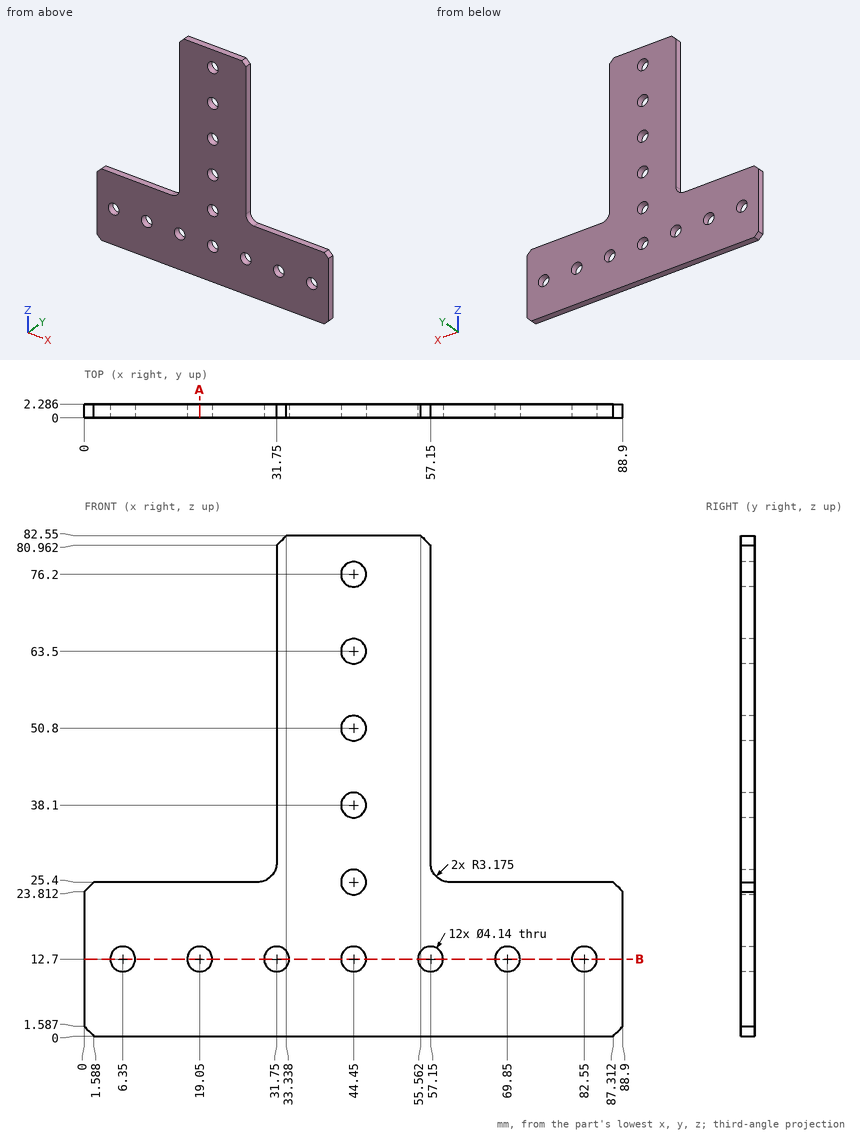
The drawing under review shows one solid part. Ordinate dimensions are in mm from its lowest x, y, z. Give positions to 0.01 mm unless a question says otherwise; leave off trailing zeros. Loops run counter-clockwise (first coordinate to the right, second up) from the corner with the lowest first, then second, coordinate; pieces in that order, holes last. Notation, with made-up numbers: M -4.75,-18 L 12.25,-18 A13 ccw 12.25,1 Z; hole C 47.25,-21 d8. An arc over 180 degrees is marked long. One line per item, written item: value. Start each with the question number.
Q1. Add section B-B (z = 12.7). Count the separate pieces of the cut face and the enclosed holes in it, and give its area (3 significant figures).
Q2. For L1, parallel to X at y = 0.6, z = 63.5; L2, parallel to Z at x = 25.5, y = 1.2; L3, parallel to Z at x = 56, y = 1.4 (1 decimal), list the stretches that pass through material, from the lowest coordinate up.
Q3. Add section A-A (x = 19.05). Give the boundary of the cut face in (y, z) (1 decimal).
Q4. Clearance check with flat-ended pins moving along their axes: pin 1 Ø5.5 at (x, z) = (44.45, 12.7) entering from -Y; pin 2 Ø3.5 at (x, z) = (82.55, 12.7) entering from -Y; pin 3 Ø0.7 at (y, z) = (1.5, 42) entering from -X; pin 4 Ø0.7 at (y, z) = (1.5, 54.5) entering from +X. State where each tip first meets the part, or that it passes through.
Reply:
1. separate pieces: 8
1. enclosed holes: 0
1. area: 137 mm²
2. L1: 31.75 to 42.38, 46.52 to 57.15
2. L2: 0 to 25.4
2. L3: 0 to 11, 14.4 to 82.1
3. outline: M 0,0 L 2.3,0 L 2.3,10.6 L 0,10.6 Z; M 0,14.8 L 2.3,14.8 L 2.3,25.4 L 0,25.4 Z
4. pin 1: y = 0
4. pin 2: through
4. pin 3: x = 31.75
4. pin 4: x = 57.15
